Verification items for the finished model (mm, model axes). A direction names the side the tool comes from. Coordinates: 2 decimals unless noted, no trailing zeros. Loops run counter-clockwise (first coordinate to the right, second up) from the corner with the lowest first, then second, coordinate; pieces in that order, holes last. Notation, with made-up numbers: (25, 43) - (72, 43) arc R21 cw to (72, 67) - close; hole circle Ø5 at (87.5, 20.5). An arc over 180 degrees is marked (long way). Answer as CSV lines item,"result". Start each with the question number.
1. Cross-section at D-D (x = 6.5). Enter the section's corners in (y, z), plus the area to 3 significant figures.
2. Cross-section at C-C (z = 1.45). Enter the section's corners in (x, y), plus the area to 3 significant figures.
3. Material ranges on line 1 (Z direction, x = 4.75, y = 1.75); line 2 (Z direction, x = 1, y = 4.75); line 3 (X direction, y = 4, z = 3.4), recorded low to high. Write a range as [from, to].
4. Cross-section at A-A (y = 1.5). Enter the section's corners in (x, z).
5. Set-up check for faces 5 (the flat face through (3.7, 2.8, 5.8)), 6 (the flat face through (0.5, 4, 3)): record each of +Z, -Z, +X, -X, +Y, -Y from which the full face is reachable in a straight line by a thin tool's end or side.
6. Gauge pin test, flat ends, axial feed: P1, Ø0.7, axis at y = -1.5, z = 3.5, coming from the +X side; P2, Ø2.5, axis at x = 4, z = 4, coming from the +Y side; P3, Ø1, axis at x = 6, z = 4, coming from the -Y side. Record the tip position at first contact, or that the pin passes through.
7. Release check for a two-part mould opening along X. For faces 1 (the flat face through (7, 0, 3)), 2 (the flat face through (0, 4, 3)), 3 (the flat face through (5, 0.5, 2.9)), 4 (the flat face through (4, 1, 3)) record: pulls with the +X half, pulls with the -X half, needs draft (parallel to the pull), parting line crosses it, or undercut.
8. Cross-section at B-B (y = -0.75). Enter the section's corners in (x, z).
```python
from build123d import *

# Parameters (mm, degrees)
EXTRUDE_1_DEPTH      = 5.8
SKETCH_2_W           = 6.5
SKETCH_2_H           = 4.8
CUT_EXTRUDE_1_DEPTH  = 6
SKETCH_3_W           = 0.6
SKETCH_3_H           = 0.6
EXTRUDE_2_DEPTH      = 2.4
EXTRUDE_2_DEPTH_BACK = 6.1
SKETCH_5_W           = 4.5
SKETCH_5_H           = 4
CUT_EXTRUDE_2_DEPTH  = 1


with BuildPart() as part:
    # 草图1 → 凸台-拉伸1 (new body)
    with BuildSketch(Plane.XY):
        Polygon((1.5, 0), (1.5, 0.5), (3.5, 0.5), (3.5, 0), (4, 0), (4, 0.5), (6, 0.5), (6, 0), (7.5, 0), (7.5, 7), (0, 7), (0, 0), align=None)
    extrude(amount=EXTRUDE_1_DEPTH)

    # 草图2 → 切除-拉伸1 (cut)
    with BuildSketch(Plane(origin=(0, 7, 0), x_dir=(1, 0, 0), z_dir=(0, 1, 0))):
        with Locations((3.75, -2.9)):
            Rectangle(SKETCH_2_W, SKETCH_2_H)
    extrude(amount=-CUT_EXTRUDE_1_DEPTH, mode=Mode.SUBTRACT)

    # 草图3 → 凸台-拉伸2 (add, two sides)
    with BuildSketch(Plane.XZ) as extrude_2_sk:
        with Locations((2.5, 3.4)):
            Rectangle(SKETCH_3_W, SKETCH_3_H)
        with Locations((5, 3.4)):
            Rectangle(SKETCH_3_W, SKETCH_3_H)
    extrude(amount=EXTRUDE_2_DEPTH)
    extrude(extrude_2_sk.sketch, amount=-EXTRUDE_2_DEPTH_BACK)

    # 草图5 → 切除-拉伸2 (cut)
    with BuildSketch(Plane.XY.offset(5.8)):
        with Locations((3.75, 5)):
            Rectangle(SKETCH_5_W, SKETCH_5_H)
    extrude(amount=-CUT_EXTRUDE_2_DEPTH, mode=Mode.SUBTRACT)


solid = part.part
```
Values follow:
1,outline,"(0, 0) - (7, 0) - (7, 0.5) - (1, 0.5) - (1, 5.3) - (7, 5.3) - (7, 5.8) - (0, 5.8) - close"
1,area,"11.8 mm²"
2,outline,"(0, 0) - (1.5, 0) - (1.5, 0.5) - (3.5, 0.5) - (3.5, 0) - (4, 0) - (4, 0.5) - (6, 0.5) - (6, 0) - (7.5, 0) - (7.5, 7) - (7, 7) - (7, 1) - (0.5, 1) - (0.5, 7) - (0, 7) - close"
2,area,"11.5 mm²"
3,line 1,"z = [0, 0.5], [3.1, 3.7], [5.3, 5.8]"
3,line 2,"z = [0, 0.5], [5.3, 5.8]"
3,line 3,"x = [0, 0.5], [2.2, 2.8], [4.7, 5.3], [7, 7.5]"
4,outline,"(0, 0) - (7.5, 0) - (7.5, 5.8) - (0, 5.8) - close; (2.2, 3.1) - (2.8, 3.1) - (2.8, 3.7) - (2.2, 3.7) - close; (4.7, 3.1) - (5.3, 3.1) - (5.3, 3.7) - (4.7, 3.7) - close; hole (0.5, 0.5) - (7, 0.5) - (7, 5.3) - (0.5, 5.3) - close"
5,face 5,"+Z, +X, -X, +Y, -Y"
5,face 6,"+Y"
6,P1,"stops at x = 5.3"
6,P2,"stops at y = 6.1"
6,P3,"stops at y = 0"
7,face 1,"needs draft"
7,face 2,"pulls with the -X half"
7,face 3,"undercut"
7,face 4,"undercut"
8,outline,"(2.2, 3.1) - (2.8, 3.1) - (2.8, 3.7) - (2.2, 3.7) - close; (4.7, 3.1) - (5.3, 3.1) - (5.3, 3.7) - (4.7, 3.7) - close"
